from build123d import *

# Parameters (mm, degrees)
F0_W     = 94
F0_H     = 94
F1_DEPTH = 3
F2_W     = 45
F2_H     = 15
F3_DEPTH = 3
F4_R     = 2.5796875
F5_DEPTH = 3.001
F6_R     = 5.159375
F7_DEPTH = 1.5875
F8_R     = 1
F9_DEPTH = 18.001


# Not quite as in the source:
# - a length typed as a fraction of an inch, garbled in the dataset ("3 / 203.2 mm" for 3/8 in), is restored


with BuildPart() as f1:
    # F0 (on Front) → F1 (new body)
    with BuildSketch(Plane.XZ):
        Rectangle(F0_W, F0_H)
    extrude(amount=F1_DEPTH)

    # F2 (on face) → F3 (join)
    with BuildSketch(Plane(origin=(0, 0, -47), x_dir=(1, 0, 0), z_dir=(0, 0, -1))):
        with Locations((0, -7.5)):
            Rectangle(F2_W, F2_H)
    extrude(amount=-F3_DEPTH)

    # F4 (on face) → F5 (cut, through all)
    with BuildSketch(Plane.XY.offset(-44)):
        with Locations((-15, 6)):
            Circle(F4_R)
        with Locations((15, 6)):
            Circle(F4_R)
    extrude(amount=-F5_DEPTH, mode=Mode.SUBTRACT)

    # F6 (on face) → F7 (cut)
    with BuildSketch(Plane.XY.offset(-44)):
        with Locations((-15, 6)):
            Circle(F6_R)
        with Locations((15, 6)):
            Circle(F6_R)
    extrude(amount=-F7_DEPTH, mode=Mode.SUBTRACT)

    # F8 (on face) → F9 (cut, through all)
    with BuildSketch(Plane.XZ.offset(3)):
        with Locations((0, 47)):
            Circle(F8_R)
    extrude(amount=-F9_DEPTH, mode=Mode.SUBTRACT)


solid = f1.part
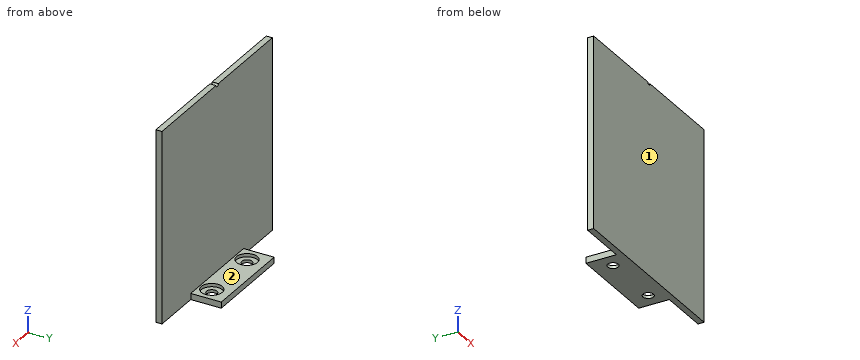
Work out the finished part from the listing and answer in its coordinate system (mm). Face numbers are marked on the shaded views. A direction names the side the tool comes from. Round coordinates to 2 decimals unless told otherwise and drop trailing zeros. Write each loop counter-clockwise with the first axis right and the second up, starting at its lowest first coordinate (ties: lowest second). Pieces come first, ordered by that corner, then holes.
1) Given pin 1 Ø3 at (x, y) = (-16.5, 7.5) entering from +Z; pin 2 Ø1 at (x, z) = (-24.5, 15) entering from +Y; pin 3 Ø1.5 at (x, y) = (-24, 8) entering from -Z; pin 4 Ø1.5 at (y, z) = (9.5, -45.5) entering from -X, each flat-ended and moving along its own axis, determine where each tip first touches the part or whether it passes through.
2) A cutting plane is placed at A-A (y = 6). Give the vertices of the cut face in (x, z), plus the area to 3 significant figures.
3) A cutting plane is placed at B-B (x = 15). Give the vertices of the cut face in (y, z).
4) A cutting plane is placed at D-D (x = -5). Give the vertices of the cut face in (y, z).
5) A cutting plane is placed at C-C (z = -40). Give the vertices of the cut face in (x, y), plus the area to 3 significant figures.
6) Straight lines are drawn through the part: line 1 (Y direction, x = -15, z = -44.35); line 2 (Y direction, x = 15, z = -46.5); line 3 (Y direction, x = 13.5, z = 10.5). For each, find the intervals that lie inside material, in ascending order.
7) A tool of negligible diameter and unlimited length cuts with its end or side. For the marked faces 1 and 2, from which of +Z, -Z, +X, -X, +Y, -Y can it reach the whole face along a straight path? Write none if from no direction.
Completed:
1. pin 1: stops at z = -45.59
1. pin 2: stops at y = 0
1. pin 3: passes through
1. pin 4: stops at x = -22.5
2. outline: (-22.5, -47) - (-17.58, -47) - (-17.58, -45.59) - (-20.16, -45.59) - (-20.16, -44) - (-22.5, -44) - close; (-12.42, -47) - (12.42, -47) - (12.42, -45.59) - (9.84, -45.59) - (9.84, -44) - (-9.84, -44) - (-9.84, -45.59) - (-12.42, -45.59) - close; (17.58, -47) - (22.5, -47) - (22.5, -44) - (20.16, -44) - (20.16, -45.59) - (17.58, -45.59) - close
2. area: 87.7 mm2
3. outline: (-3, -47) - (3.42, -47) - (3.42, -45.59) - (0.84, -45.59) - (0.84, -44) - (0, -44) - (0, 47) - (-3, 47) - close; (8.58, -47) - (15, -47) - (15, -44) - (11.16, -44) - (11.16, -45.59) - (8.58, -45.59) - close
4. outline: (-3, -47) - (15, -47) - (15, -44) - (0, -44) - (0, 47) - (-3, 47) - close
5. outline: (-47, -3) - (47, -3) - (47, 0) - (-47, 0) - close
5. area: 282 mm2
6. line 1: y = -3 to 0.84, 11.16 to 15
6. line 2: y = -3 to 3.42, 8.58 to 15
6. line 3: y = -3 to 0
7. face 1: +Z, -Z, +X, -X, -Y
7. face 2: +Z, +X, -X, +Y
